Geometry: final body of the model. Coordinates: model frame, mm. A direction names the side the tool comes from. Coordinates: 2 decimals unless noted, no trailing zeros. Write each loop counter-clockwise with the first axis right and the second up, starting at its lowest first coordinate (ties: lowest second). Pieces come first, ordered by that corner, then holes. Notation, with made-up numbers: (20.25, 21) - (27.25, 21) arc R16 cw to (27.25, 25) - close; hole circle Ø11 at (-38.5, 16). An arc over 180 degrees is marked (long way). Put each result on its own line as item: value.
```python
from build123d import *

# Parameters (mm, degrees)
PAD_DEPTH               = 35
POCKET_DEPTH            = 25
SKETCH002_W             = 6.4
SKETCH002_H             = 2.5
PAD001_DEPTH            = 9
SKETCH003_R             = 1.55
PAD002_DEPTH            = 9
PAD003_DEPTH            = 33
SKETCH002_MIRRORED_2_W  = 6.4
SKETCH002_MIRRORED_2_H  = 2.5
PAD001_MIRRORED_2_DEPTH = 9
PAD003_MIRRORED_2_DEPTH = 33
SKETCH003_MIRRORED_2_R  = 1.55
PAD002_MIRRORED_2_DEPTH = 9
POCKET001_DEPTH         = 10
PAD004_DEPTH            = 7
POCKET002_DEPTH         = 10
SKETCH008_W             = 19.5
SKETCH008_H             = 6
SKETCH009_R             = 2.85
POCKET003_DEPTH         = 0.001
POCKET003_DEPTH_BACK    = -35.001
FILLET_R                = 4


with BuildPart() as part:
    # Sketch → Pad (new body)
    with BuildSketch(Plane.XY):
        with BuildLine():
            Line((-22.6, 30.6), (22.6, 30.6))
            ThreePointArc((30.6, 22.6), (28.256854, 28.256854), (22.6, 30.6))
            Line((30.6, 22.6), (30.6, -22.6))
            ThreePointArc((22.6, -30.6), (28.256854, -28.256854), (30.6, -22.6))
            Line((22.6, -30.6), (-22.6, -30.6))
            ThreePointArc((-30.6, -22.6), (-28.256854, -28.256854), (-22.6, -30.6))
            Line((-30.6, -22.6), (-30.6, 22.6))
            ThreePointArc((-22.6, 30.6), (-28.256854, 28.256854), (-30.6, 22.6))
        make_face()
    extrude(amount=PAD_DEPTH)

    # Sketch001 → Pocket (cut)
    with BuildSketch(Plane.XY):
        with BuildLine():
            Line((-22.6, 28.3), (22.6, 28.3))
            ThreePointArc((28.3, 22.6), (26.630509, 26.630509), (22.6, 28.3))
            Line((28.3, 22.6), (28.3, -22.6))
            ThreePointArc((22.6, -28.3), (26.630509, -26.630509), (28.3, -22.6))
            Line((22.6, -28.3), (-22.6, -28.3))
            ThreePointArc((-28.3, -22.6), (-26.630509, -26.630509), (-22.6, -28.3))
            Line((-28.3, -22.6), (-28.3, 22.6))
            ThreePointArc((-22.6, 28.3), (-26.630509, 26.630509), (-28.3, 22.6))
        make_face()
    extrude(amount=POCKET_DEPTH, mode=Mode.SUBTRACT)

    # Sketch002 → Pad001 (join)
    with BuildSketch(Plane.XY):
        with Locations((16.3, 27.35)):
            Rectangle(SKETCH002_W, SKETCH002_H)
    pad001 = extrude(amount=PAD001_DEPTH)

    # Sketch003 → Pad002 (join)
    with BuildSketch(Plane.XY):
        with Locations((28.1, 15.6)):
            Circle(SKETCH003_R)
    pad002 = extrude(amount=PAD002_DEPTH)

    # Sketch004 → Pad003 (join)
    with BuildSketch(Plane.XY):
        with BuildLine():
            Line((21.8, 3.3), (12.7, 3.3))
            Line((12.7, 3.3), (12.7, 5.5))
            ThreePointArc((14.7, 7.5), (13.285786, 6.914214), (12.7, 5.5))
            Line((14.7, 7.5), (19.8, 7.5))
            ThreePointArc((21.8, 5.5), (21.214214, 6.914214), (19.8, 7.5))
            Line((21.8, 5.5), (21.8, 3.3))
        make_face()
    pad003 = extrude(amount=PAD003_DEPTH)

    # Sketch002 Mirrored 2 → Pad001 Mirrored 2 (add)
    with BuildSketch(Plane(origin=(0, 0, 0), x_dir=(-1, 0, 0), z_dir=(0, 0, -1))):
        with Locations((16.3, 27.35)):
            Rectangle(SKETCH002_MIRRORED_2_W, SKETCH002_MIRRORED_2_H)
    pad001_mirrored_2 = extrude(amount=-PAD001_MIRRORED_2_DEPTH)

    # Sketch004 Mirrored 2 → Pad003 Mirrored 2 (add)
    with BuildSketch(Plane(origin=(0, 0, 0), x_dir=(-1, 0, 0), z_dir=(0, 0, -1))):
        with BuildLine():
            Line((21.8, 3.3), (12.7, 3.3))
            Line((12.7, 3.3), (12.7, 5.5))
            ThreePointArc((14.7, 7.5), (13.285786, 6.914214), (12.7, 5.5))
            Line((14.7, 7.5), (19.8, 7.5))
            ThreePointArc((21.8, 5.5), (21.214214, 6.914214), (19.8, 7.5))
            Line((21.8, 5.5), (21.8, 3.3))
        make_face()
    pad003_mirrored_2 = extrude(amount=-PAD003_MIRRORED_2_DEPTH)

    # Sketch003 Mirrored 2 → Pad002 Mirrored 2 (add)
    with BuildSketch(Plane(origin=(0, 0, 0), x_dir=(-1, 0, 0), z_dir=(0, 0, -1))):
        with Locations((28.1, 15.6)):
            Circle(SKETCH003_MIRRORED_2_R)
    pad002_mirrored_2 = extrude(amount=-PAD002_MIRRORED_2_DEPTH)

    # Mirrored001: Pad001, Pad003, Pad002, Pad001 Mirrored 2, Pad003 Mirrored 2, Pad002 Mirrored 2 across XZ
    add(pad001.mirror(Plane.XZ))
    add(pad003.mirror(Plane.XZ))
    add(pad002.mirror(Plane.XZ))
    add(pad001_mirrored_2.mirror(Plane.XZ))
    add(pad003_mirrored_2.mirror(Plane.XZ))
    add(pad002_mirrored_2.mirror(Plane.XZ))

    # Sketch005 → Pocket001 (cut, symmetric)
    with BuildSketch(Plane.XZ):
        Polygon((-12.75, 1), (12.75, 1), (17.5, 0), (-17.5, 0), align=None)
    extrude(amount=POCKET001_DEPTH, both=True, mode=Mode.SUBTRACT)

    # Sketch006 → Pad004 (join)
    with BuildSketch(Plane.XY.offset(2)):
        with BuildLine():
            Line((23.95, 5), (12.95, 5))
            Line((12.95, 5), (12.95, -5))
            Line((12.95, -5), (23.95, -5))
            Line((23.95, -5), (23.95, -2.25))
            Line((19, -2.25), (23.95, -2.25))
            ThreePointArc((19, 2.25), (16.75, 0), (19, -2.25))
            Line((19, 2.25), (23.95, 2.25))
            Line((23.95, 2.25), (23.95, 5))
        make_face()
    pad004 = extrude(amount=PAD004_DEPTH)

    # Sketch007 → Pocket002 (cut)
    with BuildSketch(Plane.XY.offset(9)):
        with BuildLine():
            ThreePointArc((19, 5), (14, 0), (19, -5))
            Line((19, -5), (25, -5))
            Line((25, 5), (25, -5))
            Line((19, 5), (25, 5))
        make_face()
    pocket002 = extrude(amount=POCKET002_DEPTH, mode=Mode.SUBTRACT)

    # Mirrored002: Pad004, Pocket002 across YZ
    add(pad004.mirror(Plane.YZ))
    add(pocket002.mirror(Plane.YZ), mode=Mode.SUBTRACT)

    # Sketch008 → Groove (revolve, cut)
    with BuildSketch(Plane.XZ):
        with Locations((9.75, 32)):
            Rectangle(SKETCH008_W, SKETCH008_H)
    revolve(axis=Axis((0, 0, 0), (0, 0, 1)), mode=Mode.SUBTRACT)

    # Sketch009 → Pocket003 (cut, two sides)
    with BuildSketch(Plane.XY) as pocket003_sk:
        with Locations((9.5, 0)):
            Circle(SKETCH009_R)
        with Locations((-9.5, 0)):
            Circle(SKETCH009_R)
    extrude(amount=-POCKET003_DEPTH, mode=Mode.SUBTRACT)
    extrude(pocket003_sk.sketch, amount=-POCKET003_DEPTH_BACK, mode=Mode.SUBTRACT)

    # Fillet
    fillet_edges = [part.edges().sort_by_distance(p)[0] for p in [
        (0, -30.6, 35),
    ]]
    fillet(fillet_edges, radius=FILLET_R)


solid = part.part
```
1. Ray query, probe 1 along Y at (x, z) = (22.5, 5); probe 2 along X at (y, z) = (0, 27); probe 3 along X at (y, z) = (-5.5, 14). Return the intervals inside material, ascending. Write a range as from..to.
Answer below:
probe 1: y = -30.6..-28.3, -5..-2.25, 2.25..5, 28.3..30.6
probe 2: x = -30.6..-12.35, -6.65..6.65, 12.35..30.6
probe 3: x = -30.6..-28.3, -21.8..-12.7, 12.7..21.8, 28.3..30.6
2. Mould query, pull axis X, two halves, no side actions, for faces 1 (the flat face through (30.6, 0, 15)), 2 (the flat face through (-13.1, -27, 4)), 3 (the flat face through (20, 5, 0)), 4 (the flat face through (-30.6, 0, 15)). Classes: +X half, -X half, draft (parallel to the pull), parting line (faces both ways), or undercut.
Answer below:
face 1: +X half
face 2: undercut
face 3: draft
face 4: -X half
3. Pin query (flat end, axial travel): pin 1 Ø5 at (x, y) = (-22.5, -1) entering from -Z; pin 2 Ø1.4 at (x, y) = (27.5, -15) entering from +Z (3 decimals); pin 3 Ø6.5 at (x, y) = (9.5, 0) entering from -Z; pin 4 Ø0.7 at (y, z) = (-27, 6) entering from +X. Return the tip coordinate at first contact, or that it passes through.
Answer below:
pin 1: stops at z = 0
pin 2: stops at z = 34.995
pin 3: stops at z = 25
pin 4: stops at x = 29.5
4. Section query C-C (x = 0). Return loops of the section in (y, z), then the cut area to 3 significant figures.
Answer below:
outline: (-30.6, 0) - (-28.3, 0) - (-28.3, 25) - (28.3, 25) - (28.3, 0) - (30.6, 0) - (30.6, 31) arc R4 ccw to (26.6, 35) - (19.5, 35) - (19.5, 29) - (-19.5, 29) - (-19.5, 35) - (-26.6, 35) arc R4 ccw to (-30.6, 31) - close
area: 486 mm²
5. Section query D-D (z = 16). Count the separate pieces of the cut face and the enclosed holes in it, then the cut area to 3 significant figures.
Answer below:
separate pieces: 5
enclosed holes: 1
area: 624 mm²
6. Set-up query: faces 5 (the flat face through (-20, -5, 14)), 6 (the flat face through (20, -5, 0)), 7 (the cylindrical face through (26.59, -26.67, 12.32)). Return all of +Z, -Z, +X, -X, +Y, -Y with unobstructed straight access to the full face (end or side cutting, diameter ignored); none if empty.
Answer below:
face 5: none
face 6: -Z, +X, -X, +Y, -Y
face 7: -Z
7. Section query A-A (x = 9.5). Return loops of the section in (y, z), then the cut area to 3 significant figures.
Answer below:
outline: (-30.6, 0) - (-28.3, 0) - (-28.3, 25) - (-2.85, 25) - (-2.85, 29) - (-17.03, 29) - (-17.03, 35) - (-26.6, 35) arc R4 ccw to (-30.6, 31) - close; (2.85, 25) - (28.3, 25) - (28.3, 0) - (30.6, 0) - (30.6, 31) arc R4 ccw to (26.6, 35) - (17.03, 35) - (17.03, 29) - (2.85, 29) - close
area: 493 mm²
8. Section query B-B (y = 15.6). Return loops of the section in (x, z).
Answer below:
outline: (-30.6, 0) - (-26.55, 0) - (-26.55, 9) - (-28.3, 9) - (-28.3, 25) - (28.3, 25) - (28.3, 9) - (26.55, 9) - (26.55, 0) - (30.6, 0) - (30.6, 31) arc R4 ccw to (26.6, 35) - (11.7, 35) - (11.7, 29) - (-11.7, 29) - (-11.7, 35) - (-26.6, 35) arc R4 ccw to (-30.6, 31) - close
